Here's how the part is built. I have some questions about the finished solid (model axes, mm). Face numbers are marked on the shaded views. A direction names the side the tool comes from. Round coordinates to 2 decimals unless told otherwise and drop trailing zeros. Loops run counter-clockwise (first coordinate to the right, second up) from the corner with the lowest first, then second, coordinate; pieces in that order, holes last. Notation, with made-up numbers: (-6, -13.75) -> (26, -13.75) arc R14 ccw to (26, 1.25) -> close; hole circle Ø10 at (17, -12.75). An arc over 180 degrees is marked (long way). Use one line per item in the form item = value. Start each with the question number.
Item 1: If I drill on L1, parallel to X at y = 38, z = 28.5; L2, parallel to Y at x = -22.5, z = 59; L3, parallel to Z at x = 94, y = -26, over which ranges is the centre line in solid material (lowest first)? Write a range as [from, to].
Item 2: I'm going to push a flat-ended pin straight in: pin 1 Ø2 at (x, z) = (-75.5, 115) entering from -Y. Where does the tip first touch, or does it pass through?
Item 3: If we section it at B-B (z = 106): Write out the boundary of the cut face in (x, y).
Item 4: If we section it at C-C (y = -39.5): Write out the boundary of the cut face in (x, z).
Item 5: If we section it at D-D (x = -38): Write out the boundary of the cut face in (y, z).
Item 6: Thinking about a two-plate mould opening in Y: for the marked faces 3, 4, 5 and 6, which applies, released by +Y, released by -Y, zero draft, split by the parting line, or undercut?
Item 7: For the marked faces 1 and 2, which set-ups out of +Z, -Z, +X, -X, +Y, -Y let a thin tool reach every point of the face, with its end or its side?
Item 8: If we section it at A-A (y = 55.25): Write out the boundary of the cut face in (x, z).
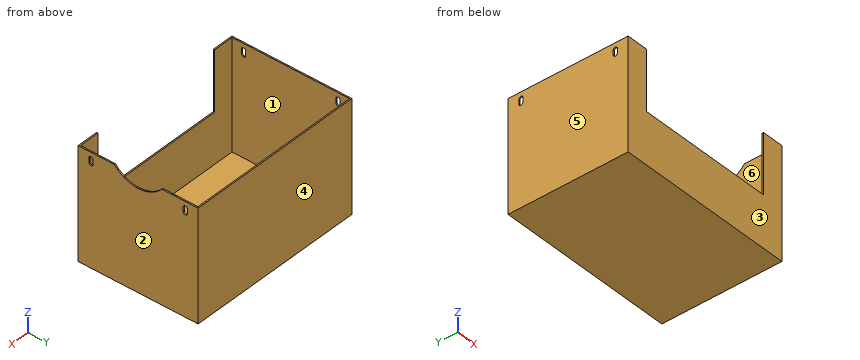
```python
from build123d import *

# Parameters (mm, degrees)
SKETCH_1_W               = 210.5
SKETCH_1_H               = 140.5
EXTRUDE_1_DEPTH          = 130
SHELL_1_T                = -1.5
CUT_EXTRUDE_2_REACH      = 259.187
CUT_EXTRUDE_3_REACH      = 220.444
SKETCH_3_W               = 160
SKETCH_3_H               = 70
CUT_EXTRUDE_4_DEPTH      = 258.187310146
CUT_EXTRUDE_4_DEPTH_BACK = 258.187310146


with BuildPart() as part:
    # 草图1 → 凸台-拉伸1 (new body)
    with BuildSketch(Plane.XY):
        Rectangle(SKETCH_1_W, SKETCH_1_H)
    extrude(amount=EXTRUDE_1_DEPTH)

    # 抽壳1
    shell_1_openings = [part.faces().sort_by_distance(p)[0] for p in [
        (0, 0, 130),
    ]]
    offset(amount=SHELL_1_T, openings=shell_1_openings, kind=Kind.INTERSECTION)

    # 草图2 → 切除-拉伸2 (cut, up to next)
    with BuildSketch(Plane(origin=(105.25, 0, 0), x_dir=(0, 0, -1), z_dir=(1, 0, 0)), mode=Mode.PRIVATE) as cut_extrude_2_sk1:
        with BuildLine():
            Line((-130, 27.694764848), (-130, -27.694764848))
            ThreePointArc((-130, -27.694764848), (-117, 0), (-130, 27.694764848))
        make_face()
    cut_extrude_2_tool1 = extrude(cut_extrude_2_sk1.sketch, amount=-CUT_EXTRUDE_2_REACH, mode=Mode.PRIVATE) & part.part
    add(cut_extrude_2_tool1.solids().sort_by_distance((105.25, 0, 124.710058))[0], mode=Mode.SUBTRACT)

    # 草图3 → 切除-拉伸3 (cut, up to next)
    with BuildSketch(Plane.XZ.offset(70.25), mode=Mode.PRIVATE) as cut_extrude_3_sk1:
        with Locations((0, 95)):
            Rectangle(SKETCH_3_W, SKETCH_3_H)
    cut_extrude_3_tool1 = extrude(cut_extrude_3_sk1.sketch, amount=-CUT_EXTRUDE_3_REACH, mode=Mode.PRIVATE) & part.part
    add(cut_extrude_3_tool1.solids().sort_by_distance((0, -70.25, 95))[0], mode=Mode.SUBTRACT)

    # 草图4 → 切除-拉伸4 (cut, two sides: drawn at the far end of the back side and taken through both)
    with BuildSketch(Plane(origin=(105.25, 0, 0), x_dir=(0, 0, -1), z_dir=(1, 0, 0)).offset(-CUT_EXTRUDE_4_DEPTH_BACK)):
        with BuildLine():
            Line((-122.5, 57.75), (-117.5, 57.75))
            ThreePointArc((-117.5, 57.75), (-115, 55.25), (-117.5, 52.75))
            Line((-117.5, 52.75), (-122.5, 52.75))
            ThreePointArc((-122.5, 52.75), (-125, 55.25), (-122.5, 57.75))
        make_face()
        with BuildLine():
            Line((-122.5, -57.75), (-117.5, -57.75))
            ThreePointArc((-117.5, -57.75), (-115, -55.25), (-117.5, -52.75))
            Line((-117.5, -52.75), (-122.5, -52.75))
            ThreePointArc((-122.5, -52.75), (-125, -55.25), (-122.5, -57.75))
        make_face()
    extrude(amount=CUT_EXTRUDE_4_DEPTH + CUT_EXTRUDE_4_DEPTH_BACK, mode=Mode.SUBTRACT)


solid = part.part
```
Values found:
q1.L1 = [-105.25, -103.75], [103.75, 105.25]
q1.L2 = [-70.25, -68.75], [68.75, 70.25]
q1.L3 = [0, 1.5]
q2.pin_1 = 68.75
q3.outline = (-105.25, -70.25) -> (-80, -70.25) -> (-80, -68.75) -> (-103.75, -68.75) -> (-103.75, 68.75) -> (103.75, 68.75) -> (103.75, -68.75) -> (80, -68.75) -> (80, -70.25) -> (105.25, -70.25) -> (105.25, 70.25) -> (-105.25, 70.25) -> close
q4.outline = (-105.25, 0) -> (105.25, 0) -> (105.25, 130) -> (103.75, 130) -> (103.75, 1.5) -> (-103.75, 1.5) -> (-103.75, 130) -> (-105.25, 130) -> close
q5.outline = (-70.25, 0) -> (70.25, 0) -> (70.25, 130) -> (68.75, 130) -> (68.75, 1.5) -> (-68.75, 1.5) -> (-68.75, 60) -> (-70.25, 60) -> close
q6.face_3 = released by -Y
q6.face_4 = released by +Y
q6.face_5 = zero draft
q6.face_6 = undercut
q7.face_1 = +Z
q7.face_2 = +Z, -Z, +X, +Y, -Y
q8.outline = (-105.25, 0) -> (105.25, 0) -> (105.25, 115) -> (103.75, 115) -> (103.75, 1.5) -> (-103.75, 1.5) -> (-103.75, 115) -> (-105.25, 115) -> close; (-105.25, 125) -> (-103.75, 125) -> (-103.75, 130) -> (-105.25, 130) -> close; (103.75, 125) -> (105.25, 125) -> (105.25, 130) -> (103.75, 130) -> close
